Design review of the part shown in the three views and the two pictorial views. Dimensions are in mm from the part's minimum x, y and z. A direction names the side the tool comes from. Round coordinates to 2 decimals unless told otherwise and drop trailing zeros. Order: outer loops, then holes, each group sorted by start corner. A loop starts at its lowest first (then second) coordinate and runs counter-clockwise, first axis right, second up. Notation, with made-up numbers: (-39, -19) - (-13, -19) arc R22 ccw to (-13, -1) - close; hole circle Ø2 at (0.5, 28). An arc over 180 degrees is marked (long way). One line per question, with ' | ' between items. Start each with the question number.
Item 1: Add section D-D on x = 67. State the section outline as (y, z) points.
Item 2: Add section C-C on y = 25. State the section outline as (x, z) points.
Item 3: Insertion check: pin 1 Ø4 at (x, y) = (51.5, 7.5) entering from +Z; pin 2 Ø3 at (y, z) = (33.5, 56.5) entering from +X; pin 3 Ø12 at (x, z) = (11, 51.5) entering from -Y; pin 4 Ø7 at (y, z) = (30.2, 46.8) entering from -X. Each pin has a flat end and moves straight along its axis. Give the tip position at first contact, or say it passes through.
Item 4: For L1, parallel to Z at x = 6, y = 9.5; L2, parallel to Y at x = 3, z = 59; L3, parallel to X at y = 7.5, z = 20.5, list the stretches that pass through material, from the lowest coordinate up. Write a range as [from, to].
Item 5: Tool access review of the marked faces 1 and 2: name each direction out of +Z, -Z, +X, -X, +Y, -Y from which nothing blocks a thin tool from reaching the whole face with its end or side.
Item 6: Add section B-B on z = 46.8. State the section outline as (x, y) points.
Item 7: Add section A-A on y = 30.2. State the section outline as (x, z) points.
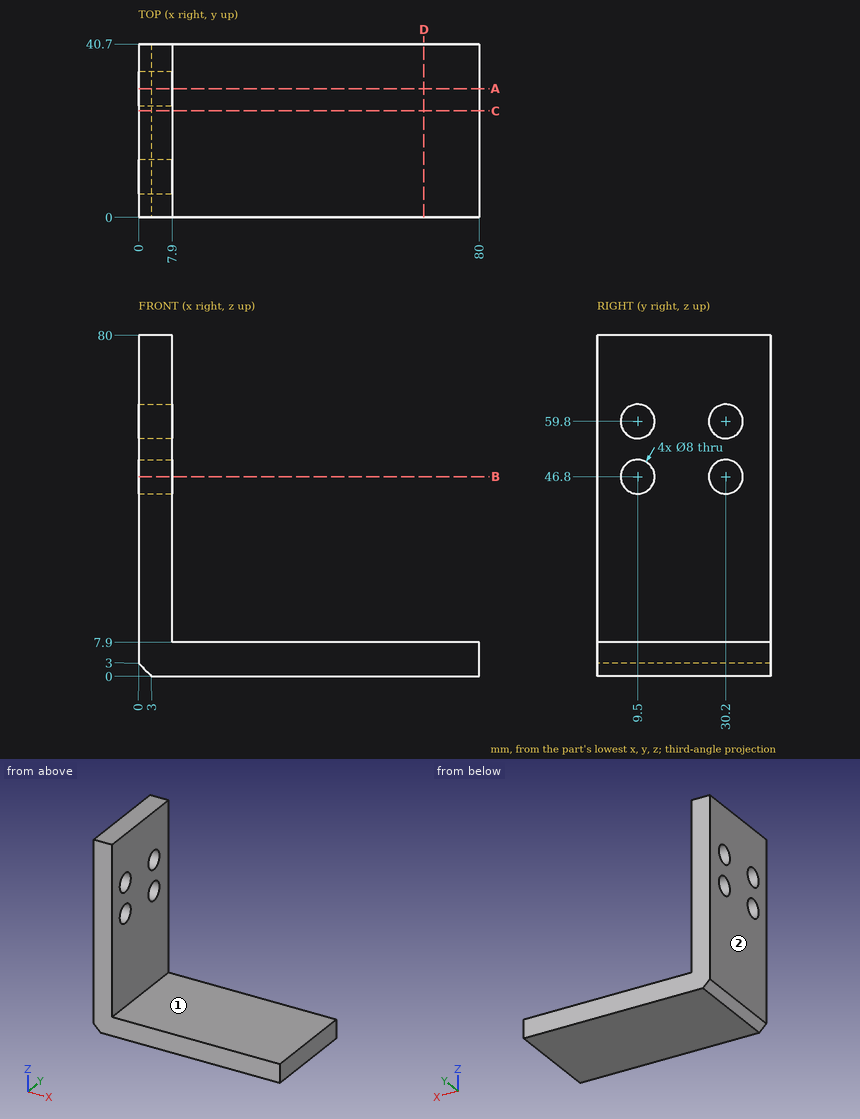
Determined:
1) outline: (0, 0) - (40.7, 0) - (40.7, 7.9) - (0, 7.9) - close
2) outline: (0, 3) - (3, 0) - (80, 0) - (80, 7.9) - (7.9, 7.9) - (7.9, 80) - (0, 80) - close
3) pin 1: z = 7.9 | pin 2: x = 7.9 | pin 3: y = 0 | pin 4: through
4) L1: [0, 42.8], [50.8, 55.8], [63.8, 80] | L2: [0, 5.58], [13.42, 26.28], [34.12, 40.7] | L3: [0, 7.9]
5) face 1: +Z, +X, +Y, -Y | face 2: +Z, -Z, -X, +Y, -Y
6) outline: (0, 0) - (7.9, 0) - (7.9, 5.5) - (0, 5.5) - close; (0, 13.5) - (7.9, 13.5) - (7.9, 26.2) - (0, 26.2) - close; (0, 34.2) - (7.9, 34.2) - (7.9, 40.7) - (0, 40.7) - close
7) outline: (0, 3) - (3, 0) - (80, 0) - (80, 7.9) - (7.9, 7.9) - (7.9, 42.8) - (0, 42.8) - close; (0, 50.8) - (7.9, 50.8) - (7.9, 55.8) - (0, 55.8) - close; (0, 63.8) - (7.9, 63.8) - (7.9, 80) - (0, 80) - close
